Autodesk Inventor part; units mm, degrees
ref_plane "YZ Plane" through (0, 0, 0) normal (1, 0, 0) x (0, 1, 0)
ref_plane "XZ Plane" through (0, 0, 0) normal (0, 1, 0) x (-1, 0, 0)
ref_plane "XY Plane" through (0, 0, 0) normal (0, 0, 1) x (1, 0, 0)
sketch "Sketch1" plane through (0, 0, 0) normal (0, 1, 0) x (-1, 0, 0)
  line L0 (1, 0) -> (49, 0)
  line L1 (50, -1) -> (50, -99)
  line L2 (49, -100) -> (1, -100)
  line L3 (0, -99) -> (0, -1)
  line L4 (50, 2) -> (0, 2)
  line L5 (-2, 0) -> (-2, -100)
  line L6 (0, -102) -> (50, -102)
  line L7 (52, -100) -> (52, 0)
  arc A0 (52, 0) -> (50, 2) centre (50, 0) ccw
  arc A1 (0, 2) -> (-2, 0) centre (0, 0) ccw
  arc A2 (-2, -100) -> (0, -102) centre (0, -100) ccw
  arc A3 (50, -102) -> (52, -100) centre (50, -100) ccw
  arc A4 (50, -1) -> (49, 0) centre (49, -1) ccw
  arc A5 (1, 0) -> (0, -1) centre (1, -1) ccw
  arc A6 (0, -99) -> (1, -100) centre (1, -99) ccw
  arc A7 (49, -100) -> (50, -99) centre (49, -99) ccw
  point P0 (0, 0)
  point P1 (50, -100)
  point P2 (50, 0)
  point P3 (0, -100)
  point P4 (-2, -102)
  point P5 (-2, 2)
  point P6 (52, -102)
  dimension "d0" = 50
  dimension "d1" = 100
  dimension "d2" = 54
  dimension "d3" = 104
  dimension "d4" = 2
  dimension "d5" = 2
  dimension "d6" = 2
  dimension "d7" = 1
extrude "Extrusion1" add sketch "Sketch1" along normal blind 4 contours L0 A4 L1 A7 L2 A6 L3 A5
extrude "Extrusion2" add sketch "Sketch1" along normal blind 2
fillet "Fillet1" radius 0.5 24 edges at (-0.2929, 4, -0.2929) (0, 4, -50) (-0.2929, 4, -99.7071) (-25, 4, -100) (-49.7071, 4, -99.7071) (-50, 4, -50) (-49.7071, 4, -0.2929) (-25, 4, 0) (1.4142, 2, 1.4142) (2, 2, -50) (1.4142, 2, -101.4142) (-25, 2, -102) (-51.4142, 2, -101.4142) (-52, 2, -50) (-51.4142, 2, 1.4142) (-25, 2, 2) (1.4142, 0, 1.4142) (2, 0, -50) (1.4142, 0, -101.4142) (-25, 0, -102) (-51.4142, 0, -101.4142) (-52, 0, -50) (-51.4142, 0, 1.4142) (-25, 0, 2)
properties part number "connection box lid"
Verification items for the finished model (mm, model axes). Coordinates: 2 decimals unless noted, no trailing zeros. Write each loop counter-clockwise with the first axis right and the second up, starting at its lowest first coordinate (ties: lowest second). Pieces come first, ordered by that corner, then holes. Notation, with made-up numbers: M -25,77.25 L -3,77.25 A13 cw -3,86.25 Z; hole C 30.25,4.5 d4. An arc over 180 degrees is marked long. Use a Markdown table: item, result.
Q1. Sectioned sample at B-B, the plane x = -21. Record the boundary of the cut face in (y, z).
Reply:
| item | result |
|---|---|
| outline | M 0,-101.5 A0.5 ccw 0.5,-102 L 1.5,-102 A0.5 ccw 2,-101.5 L 2,-100 L 3.5,-100 A0.5 ccw 4,-99.5 L 4,-0.5 A0.5 ccw 3.5,0 L 2,0 L 2,1.5 A0.5 ccw 1.5,2 L 0.5,2 A0.5 ccw 0,1.5 Z |
Q2. Sectioned sample at A-A, the plane z = -10. Record the boundary of the cut face in (x, y).
Reply:
| item | result |
|---|---|
| outline | M -52,0.5 A0.5 ccw -51.5,0 L 1.5,0 A0.5 ccw 2,0.5 L 2,1.5 A0.5 ccw 1.5,2 L 0,2 L 0,3.5 A0.5 ccw -0.5,4 L -49.5,4 A0.5 ccw -50,3.5 L -50,2 L -51.5,2 A0.5 ccw -52,1.5 Z |
Q3. Thickness scan on line 1 (Z direction, x = -16.5, y = 3.05); line 2 (X direction, y = 2.35, z = -8.5); line 3 (Z direction, x = -17.5, y = 0.25). Record the ranges inside material, lowest first.
Reply:
| item | result |
|---|---|
| line 1 | z = -100 to 0 |
| line 2 | x = -50 to 0 |
| line 3 | z = -101.93 to 1.93 |
Q4. Go/stop test with a flat-tipped pin: P1, Ø1, axis at x = -39, y = 3.5, coming from the +Z side. Record where the tip stops, or that it passes through.
Reply:
| item | result |
|---|---|
| P1 | stops at z = 0 |
